```python
from build123d import *

# Parameters (mm, degrees)
SKIZZE5_R                       = 2.85
AUFSATZ_LINEAR_AUSTRAGEN2_DEPTH = 5
SKIZZE7_R                       = 1.5
SKIZZE7_R_2                     = 2.5
SCHNITT_LINEAR_AUSTRAGEN1_DEPTH = 5
SKIZZE10_R                      = 3.4
AUFSATZ_LINEAR_AUSTRAGEN4_DEPTH = 5
SKIZZE11_R                      = 1.05
SCHNITT_LINEAR_AUSTRAGEN3_DEPTH = 5
SKIZZE15_R                      = 2.25
SCHNITT_LINEAR_AUSTRAGEN7_DEPTH = 2
SKIZZE16_W                      = 8.368883353
SKIZZE16_H                      = 55.536319394
SCHNITT_LINEAR_AUSTRAGEN8_DEPTH = 1.7
SKIZZE17_W                      = 2.331134025
SKIZZE17_H                      = 18.40252581
SKIZZE17_W_2                    = 6.80460091
SKIZZE17_H_2                    = 1.708942227
SKIZZE17_W_3                    = 9.007409032
SKIZZE17_H_3                    = 2.575965086
SKIZZE17_W_4                    = 1.92022312
SKIZZE17_H_4                    = 5.063487197
SKIZZE17_H_5                    = 4.286912164
SCHNITT_LINEAR_AUSTRAGEN9_DEPTH = 11.7


with BuildPart() as part:
    # Skizze5 → Aufsatz-Linear austragen2 (new body)
    with BuildSketch(Plane.XY):
        with BuildLine():
            Line((-40.726132402, -24.649552882), (-40.726132402, 23.890447118))
            ThreePointArc((-40.726132402, 23.890447118), (-44.126132402, 20.490447118), (-47.526132402, 23.890447118))
            Line((-47.526132402, 23.890447118), (-47.526132402, -24.649552882))
            ThreePointArc((-47.526132402, -24.649552882), (-44.126132402, -21.249552882), (-40.726132402, -24.649552882))
        make_face()
        with BuildLine():
            Line((-40.726132402, 23.890447118), (-40.775983963, 24.470537999))
            ThreePointArc((-40.775983963, 24.470537999), (-44.126132402, 27.290447118), (-47.476280842, 24.470537999))
            Line((-47.476280842, 24.470537999), (-47.526132402, 23.890447118))
            ThreePointArc((-47.526132402, 23.890447118), (-44.126132402, 20.490447118), (-40.726132402, 23.890447118))
        make_face()
        with Locations((-44.126132402, 30.290447118)):
            Circle(SKIZZE5_R)
        with BuildLine():
            Line((-40.775983963, 24.470537999), (-41.276132402, 30.290447118))
            ThreePointArc((-41.276132402, 30.290447118), (-44.126132402, 27.440447118), (-46.976132402, 30.290447118))
            Line((-46.976132402, 30.290447118), (-47.476280842, 24.470537999))
            ThreePointArc((-47.476280842, 24.470537999), (-44.126132402, 27.290447118), (-40.775983963, 24.470537999))
        make_face()
        with BuildLine():
            Line((-40.775983963, -25.229643764), (-40.726132402, -24.649552882))
            ThreePointArc((-40.726132402, -24.649552882), (-44.126132402, -21.249552882), (-47.526132402, -24.649552882))
            Line((-47.526132402, -24.649552882), (-47.476280842, -25.229643764))
            ThreePointArc((-47.476280842, -25.229643764), (-44.126132402, -28.049552882), (-40.775983963, -25.229643764))
        make_face()
        with BuildLine():
            Line((-41.276132402, -31.049552882), (-40.775983963, -25.229643764))
            ThreePointArc((-40.775983963, -25.229643764), (-44.126132402, -28.049552882), (-47.476280842, -25.229643764))
            Line((-47.476280842, -25.229643764), (-46.976132402, -31.049552882))
            ThreePointArc((-46.976132402, -31.049552882), (-44.126132402, -28.199552882), (-41.276132402, -31.049552882))
        make_face()
        with Locations((-44.126132402, -31.049552882)):
            Circle(SKIZZE5_R)
    extrude(amount=AUFSATZ_LINEAR_AUSTRAGEN2_DEPTH)

    # Skizze7 → Schnitt-Linear austragen1 (cut)
    with BuildSketch(Plane(origin=(0, 0, 0), x_dir=(-1, 0, 0), z_dir=(0, 0, -1))):
        with Locations((44.126132402, 30.290447118)):
            Circle(SKIZZE7_R)
        with Locations((44.126132402, 23.890447118)):
            Circle(SKIZZE7_R_2)
        with Locations((44.126132402, -24.649552882)):
            Circle(SKIZZE7_R_2)
        with Locations((44.126132402, -31.049552882)):
            Circle(SKIZZE7_R)
    extrude(amount=-SCHNITT_LINEAR_AUSTRAGEN1_DEPTH, mode=Mode.SUBTRACT)

    # Skizze10 → Aufsatz-Linear austragen4 (add)
    with BuildSketch(Plane(origin=(0, 0, 0), x_dir=(-1, 0, 0), z_dir=(0, 0, -1))):
        with Locations((44.126132402, 23.890447118)):
            Circle(SKIZZE10_R)
        with Locations((44.126132402, -24.649552882)):
            Circle(SKIZZE10_R)
    extrude(amount=-AUFSATZ_LINEAR_AUSTRAGEN4_DEPTH)

    # Skizze11 → Schnitt-Linear austragen3 (cut)
    with BuildSketch(Plane(origin=(0, 0, 0), x_dir=(-1, 0, 0), z_dir=(0, 0, -1))):
        with Locations((44.126132402, -24.649552882)):
            Circle(SKIZZE11_R)
        with Locations((44.126132402, 23.890447118)):
            Circle(SKIZZE11_R)
    extrude(amount=-SCHNITT_LINEAR_AUSTRAGEN3_DEPTH, mode=Mode.SUBTRACT)

    # Skizze15 → Schnitt-Linear austragen7 (cut)
    with BuildSketch(Plane(origin=(0, 0, 0), x_dir=(-1, 0, 0), z_dir=(0, 0, -1))):
        with Locations((44.126132402, 30.290447118)):
            Circle(SKIZZE15_R)
        with Locations((44.126132402, -31.049552882)):
            Circle(SKIZZE15_R)
    extrude(amount=-SCHNITT_LINEAR_AUSTRAGEN7_DEPTH, mode=Mode.SUBTRACT)

    # Skizze16 → Schnitt-Linear austragen8 (cut)
    with BuildSketch(Plane.XY.offset(5)):
        with Locations((-44.250355177, -0.588324363)):
            Rectangle(SKIZZE16_W, SKIZZE16_H)
    extrude(amount=-SCHNITT_LINEAR_AUSTRAGEN8_DEPTH, mode=Mode.SUBTRACT)

    # Skizze17 → Schnitt-Linear austragen9 (cut)
    with BuildSketch(Plane(origin=(0, 0, 0), x_dir=(-1, 0, 0), z_dir=(0, 0, -1))):
        with Locations((46.36056539, -0.295648179)):
            Rectangle(SKIZZE17_W, SKIZZE17_H)
        with Locations((44.482182567, 33.645654459)):
            Rectangle(SKIZZE17_W_2, SKIZZE17_H_2)
        with Locations((44.254699543, -34.820369049)):
            Rectangle(SKIZZE17_W_3, SKIZZE17_H_3)
        with Locations((40.545518977, 29.95066177)):
            Rectangle(SKIZZE17_W_4, SKIZZE17_H_4)
        with Locations((40.545518977, -30.43359055)):
            Rectangle(SKIZZE17_W_4, SKIZZE17_H_5)
    extrude(amount=-SCHNITT_LINEAR_AUSTRAGEN9_DEPTH, mode=Mode.SUBTRACT)


solid = part.part
```
Geometry check sheet. Reference: the model listing, model coordinates, mm. A direction names the side the tool comes from. Coordinates: 2 decimals unless noted, no trailing zeros. Write each loop counter-clockwise with the first axis right and the second up, starting at its lowest first coordinate (ties: lowest second). Pieces come first, ordered by that corner, then holes. Notation, with made-up numbers: M 40,61.25 L 52,61.25 A23 ccw 52,79.25 Z; hole C 62,-7 d7. An arc over 180 degrees is marked long. Use one line per item in the form item = value. Start each with the question number.
1) Section check B-B on y = 4.5. Enter the section's corners in (x, z) (3 decimals), and give its area (3 significant figures).
2) Section check A-A on x = -44.25. State how many separate pieces and enclosed holes the cut face has, and give its area (3 significant figures).
3) Thickness scan on probe 1 along Y at (x, z) = (-42.75, 1.2); probe 2 along Y at (x, z) = (-46.75, 1.6); probe 3 along Y at (x, z) = (-42.5, 1.25). Record the ranges inside material, lowest first. Write a range as from..to.
4) Section check C-C on y = 17.5. Enter the section's corners in (x, z), and give its area (3 significant figures).
5) Set-up check for faces 5 (the flat face through (-46, -9.497, 2)), 6 (the flat face through (-44, 27.18, 4)), 7 (the cylindrical face through (-42.01, 32.2, 2.46)), 8 (the cylindrical face through (-46.27, 30.97, 0.99)), 9 (the cylindrical face through (-45.512, -31.624, 3.479)): record each of +Z, -Z, +X, -X, +Y, -Y from which the full face is reachable in a straight line by a thin tool's end or side.
6) Release check for a two-part mould opening along Y. For faces 1 (the flat face through (-47.23, -28.1, 1.91)), 2 (the flat face through (-46, -30, 5)), 3 (the cylindrical face through (-45.16, -33.05, 0.99)), 4 (the cylindrical face through (-46.57, 31.76, 2.46)) record: pulls with the +Y half, pulls with the -Y half, needs draft (parallel to the pull), parting line crosses it, or undercut.
7) Go/stop test with flat-tipped pins: pin 1 Ø4 at (x, y) = (-45.5, -22) entering from -Z; pin 2 Ø1.7 at (x, y) = (-44.13, -24.65) entering from -Z; pin 3 Ø4 at (x, y) = (-44.13, 30.29) entering from -Z; pin 4 Ø1.2 at (y, z) = (30.5, 3) entering from +X. Record where each tip stops, or that it passes through.
Responses:
q1.outline = M -45.195,0 L -40.726,0 L -40.726,3.3 L -45.195,3.3 Z
q1.area = 14.7 mm2
q2.separate_pieces = 5
q2.enclosed_holes = 0
q2.area = 188 mm2
q3.probe_1 = -33.53..-32.83, -29.27..28.51, 32.07..32.79
q3.probe_2 = -32.16..-9.5, 8.91..31.4
q3.probe_3 = -33.39..-32.6, -29.49..28.74, 31.85..32.63
q4.outline = M -47.53,0 L -40.73,0 L -40.73,3.3 L -47.53,3.3 Z
q4.area = 22.4 mm2
q5.face_5 = +Z, -Z, -X
q5.face_6 = +Z, +X, -X
q5.face_7 = +Z, -Z, +X, +Y
q5.face_8 = -Z
q5.face_9 = +Z, -Z
q6.face_1 = pulls with the -Y half
q6.face_2 = needs draft
q6.face_3 = undercut
q6.face_4 = pulls with the +Y half
q7.pin_1 = 0
q7.pin_2 = through
q7.pin_3 = 2
q7.pin_4 = -41.51
